Check sheet for the modelled part. Datum: model origin and axes. Units: mm. A direction names the side the tool comes from. Round coordinates to 2 decimals unless told otherwise and drop trailing zeros. Loops run counter-clockwise (first coordinate to the right, second up) from the corner with the lowest first, then second, coordinate; pieces in that order, holes last. Notation, with made-up numbers: M 58,11 L 85,11 A18 ccw 85,22 Z; hole C -36.75,-20 d2. An arc over 180 degrees is marked long. Write item = value, one per line. Start each with the question number.
(1) Set-up check for faces 5 (the face through (16, -2, 7)), 6 (the face through (12, -10, 3)), 7 (the face through (4, -4, -3)): record each of +Z, -Z, +X, -X, +Y, -Y from which the full face is reachable in a straight line by a thin tool's end or side.
(2) Cross-section at C-C on x = 24. Record the boundary of the cut face in (y, z).
(3) Cross-section at A-A on y = -4.5. Record the boundary of the cut face in (x, z), plus the area to 3 significant figures.
(4) Scan lines: L1, parallel to Y at x = 0, z = -5.2; L2, parallel to Z at x = -6.5, y = 21; L3, parallel to Z at x = 13, y = -12.5. Record each from-to range of solid material in increasing order. Write a range as from..to.
(5) Mould release check, pull along Z, two halves, no side actions. Record for faces 1 (the face through (-4.336, -19.524, -5.465)), 2 (the face through (-18, -10, -8)), 3 (the face through (-2.413, 0.22, 11.353)), 4 (the face through (0.45, 1.3, 8.36)): pulls with the +Z half, pulls with the -Z half, needs draft (parallel to the pull), parting line crosses it, or undercut.
(6) Cross-section at B-B on y = 16.5. Record the boundary of the cut face in (x, z).
(7) Go/stop test with flat-tipped pins: P1, Ø9, axis at x = 16, z = 6.5, coming from the +Y side; P2, Ø2, axis at x = -19, y = -18, coming from the +Z side; P3, Ø12, axis at x = -12.5, y = 8, coming from the +Z side. Record where each tip stops, or that it passes through.
Autodesk Fusion 360 part; units mm, degrees
sketch "草图1" plane through (0, 0, 0) normal (0, 0, 1) x (1, 0, 0)
  circle A0 centre (0, 0) radius 27
  circle A1 centre (0, 0) radius 20
  dimension "d1" = 54
  dimension "d2" = 40
extrude "拉伸1" add sketch "草图1" against normal blind 8
extrude "拉伸2" add sketch "草图1" against normal blind 3 contours A1
sketch "草图2" plane through (0, 0, 0) normal (0, 0, 1) x (-1, 0, 0)
  circle A0 centre (0, 0) radius 27
  line L0 (-23, -10) -> (-23, 10)
  line L1 (30, 0) -> (-47, 0) construction
  dimension "d7" = 20
  dimension "d8" = 23
ref_plane "工作平面1" through (23, 0, 0) normal (0.7071, 0, 0.7071) x (0, -1, 0)
sketch "草图3" plane through (11.5, 0, 11.5) normal (0.7071, 0, 0.7071) x (0, -1, 0)
  circle A0 centre (0, 0.2635) radius 6
  line L0 (10, 0.2635) -> (10, 16.2635)
  line L1 (10, 16.2635) -> (-10, 16.2635)
  line L2 (-10, 16.2635) -> (-10, 0.2635)
  line L3 (0, 0) -> (0, 19) construction
  arc A1 (-10, 0.2635) -> (10, 0.2635) centre (0, 0.2635) ccw
  dimension "d10" = 10
  dimension "d11" = 12
  dimension "d12" = 16
extrude "拉伸3" add sketch "草图3" along normal up to surface end surface through (0, 0, -3) normal (0, 0, -1) offset 0
extrude "拉伸4" cut sketch "草图3" along normal up to surface contours A0 end surface through (0, 0, -3) normal (0, 0, -1) offset 0
Result:
q1.face_5 = +Z, +X, +Y, -Y
q1.face_6 = +Z, +X, -X, -Y
q1.face_7 = -Z
q2.outline = M -12.37,-8 L 12.37,-8 L 12.37,0 L -12.37,0 Z
q3.outline = M -26.62,-8 L -19.49,-8 L -19.49,-3 L -8.24,-3 L 8.88,14.12 L 5.37,17.63 L -12.26,0 L -26.62,0 Z; M 2.99,-3 L 19.49,-3 L 19.49,-8 L 26.62,-8 L 26.62,0 L 23,0 L 14.49,8.51 Z
q3.area = 381 mm^2
q4.L1 = -27..-20, 20..27
q4.L2 = -8..0
q4.L3 = -3..0
q5.face_1 = needs draft
q5.face_2 = pulls with the -Z half
q5.face_3 = pulls with the +Z half
q5.face_4 = undercut
q6.outline = M -21.37,-8 L -11.3,-8 L -11.3,-3 L 11.3,-3 L 11.3,-8 L 21.37,-8 L 21.37,0 L -21.37,0 Z
q7.P1 = 10
q7.P2 = 0
q7.P3 = 4.63
